Read the model definition and answer for the solid it produces. Units are mm, in the model's axes. A direction names the side the tool comes from. Round coordinates to 2 decimals unless told otherwise and drop trailing zeros. Order: outer loops, then holes, each group sorted by start corner. A loop starts at its lowest first (then second) coordinate and runs counter-clockwise, first axis right, second up. Notation, with made-up numbers: (22, 9) -> (33, 9) arc R24 ccw to (33, 38) -> close; hole circle Ø5 at (66.25, 17). An arc over 180 degrees is marked (long way). Use a Markdown table: item, result. Add a question column.
1. For faces 4 (the face through (0.99, -9.87, 31.18)), 5 (the face through (20, -24, 28)), 6 (the face through (47, -25, 6)), determine the directions among +Z, -Z, +X, -X, +Y, -Y from which every point of the face is accessible in a straight line to the end or side of a thin tool.
2. Consider L1, parallel to Z at x = 1.45, y = -11.5; L2, parallel to Z at x = 48.6, y = -11.5; L3, parallel to Z at x = 1.6, y = -16.5. Determine where each line is inside the solid, lowest interval first. Write a range as [from, to].
3. Section D-D, the plane x = 25 is taken. Give the vertices of the cut face in (y, z).
4. Section A-A, the plane x = 18 is taken. Give the vertices of the cut face in (y, z).
5. Section C-C, the plane y = -14.25 is taken. Give the vertices of the cut face in (x, z), then the cut area to 3 significant figures.
6. The mould has two halves that part along Z. Classify faces 1 (the face through (50, -12, 28)), 2 (the face through (19.01, -24.99, 27.39)), 3 (the face through (16, -25, 0)): +Z half, -Z half, draft (parallel to the pull), parting line (faces both ways), or undercut.
7. Given pin 1 (1.7 mm diameter, centred on x = 20.05, z = 33.45, fed in from +Y); pin 2 (3.5 mm diameter, centred on y = -16.5, z = 4.5, fed in from +X); pin 3 (1.5 mm diameter, centred on y = -17.5, z = 21, fed in from -X); pin 4 (3.5 mm diameter, centred on x = 25, z = 28.5, fed in from +Y), each flat-ended and moving along its own axis, determine where each tip first touches the part or whether it passes through.
8. Section B-B, the plane z = 14.5 is taken. Give the vertices of the cut face in (x, y).
```python
from build123d import *

# Parameters (mm, degrees)
EXTRUDE_1_DEPTH     = 57
SKETCH_2_R          = 7.5
SKETCH_2_R_2        = 1.5
CUT_EXTRUDE_1_DEPTH = 27
SKETCH_3_R          = 1.5
CUT_EXTRUDE_2_DEPTH = 10
SKETCH_4_R          = 1.5
SKETCH_4_R_2        = 3
SKETCH_4_R_3        = 0.75
CUT_EXTRUDE_3_DEPTH = 10
SKETCH_5_R          = 1.5
CUT_EXTRUDE_4_DEPTH = 3
FILLET_2_R          = 2
SKETCH_6_W          = 3
SKETCH_6_H          = 8
CUT_EXTRUDE_5_DEPTH = 44
FILLET_3_R          = 5


with BuildPart() as part:
    # 草图1 → 凸台-拉伸1 (new body)
    with BuildSketch(Plane.XY):
        Polygon((0, 0), (0, -26), (50, -26), (50, 0), (48, 0), (48, -24), (2, -24), (2, 0), align=None)
    extrude(amount=EXTRUDE_1_DEPTH)

    # 草图2 → 切除-拉伸1 (cut)
    with BuildSketch(Plane.ZY):
        with Locations(Location((38.5, -11.5, 0), (0, 0, 270))):
            Circle(SKETCH_2_R)
        with Locations(Location((14.5, -11.5, 0), (0, 0, 270))):
            Circle(SKETCH_2_R_2)
    extrude(amount=-CUT_EXTRUDE_1_DEPTH, mode=Mode.SUBTRACT)

    # 草图3 → 切除-拉伸2 (cut)
    with BuildSketch(Plane(origin=(2, 0, 0), x_dir=(0, 0, -1), z_dir=(1, 0, 0))):
        with Locations(Location((-4.5, -6.5, 0), (0, 0, 90))):
            Circle(SKETCH_3_R)
        with Locations(Location((-4.5, -16.5, 0), (0, 0, 90))):
            Circle(SKETCH_3_R)
        with Locations(Location((-52.5, -16.5, 0), (0, 0, 90))):
            Circle(SKETCH_3_R)
        with Locations(Location((-52.5, -6.5, 0), (0, 0, 90))):
            Circle(SKETCH_3_R)
    extrude(amount=-CUT_EXTRUDE_2_DEPTH, mode=Mode.SUBTRACT)

    # 草图4 → 切除-拉伸3 (cut)
    with BuildSketch(Plane(origin=(0, -24, 0), x_dir=(1, 0, 0), z_dir=(0, 1, 0))):
        with Locations(Location((18, -28.5, 0), (0, 0, 270))):
            Circle(SKETCH_4_R)
        with Locations(Location((25, -21.5, 0), (0, 0, 270))):
            Circle(SKETCH_4_R)
        with Locations(Location((32, -28.5, 0), (0, 0, 270))):
            Circle(SKETCH_4_R)
        with Locations(Location((25, -35.5, 0), (0, 0, 270))):
            Circle(SKETCH_4_R)
        with Locations(Location((25, -28.5, 0), (0, 0, 270))):
            Circle(SKETCH_4_R_2)
        with Locations(Location((20.050252532, -23.550252532, 0), (0, 0, 270))):
            Circle(SKETCH_4_R_3)
        with Locations(Location((29.949747468, -23.550252532, 0), (0, 0, 270))):
            Circle(SKETCH_4_R_3)
        with Locations(Location((29.949747468, -33.449747468, 0), (0, 0, 270))):
            Circle(SKETCH_4_R_3)
        with Locations(Location((20.050252532, -33.449747468, 0), (0, 0, 270))):
            Circle(SKETCH_4_R_3)
    extrude(amount=-CUT_EXTRUDE_3_DEPTH, mode=Mode.SUBTRACT)

    # 草图5 → 切除-拉伸4 (cut)
    with BuildSketch(Plane.ZY.offset(-48)):
        with Locations(Location((14.5, -11.5, 0), (0, 0, 270))):
            Circle(SKETCH_5_R)
        with Locations(Location((38.5, -11.5, 0), (0, 0, 270))):
            Circle(SKETCH_5_R)
    extrude(amount=-CUT_EXTRUDE_4_DEPTH, mode=Mode.SUBTRACT)

    # 圆角2
    fillet_2_edges = [part.edges().sort_by_distance(p)[0] for p in [
        (50, -26, 28.5),
        (0, -26, 28.5),
    ]]
    fillet(fillet_2_edges, radius=FILLET_2_R)

    # 草图6 → 切除-拉伸5 (cut)
    with BuildSketch(Plane.XZ.offset(26)):
        with Locations((48.5, 53)):
            Rectangle(SKETCH_6_W, SKETCH_6_H)
        with Locations((48.5, 4)):
            Rectangle(SKETCH_6_W, SKETCH_6_H)
    extrude(amount=-CUT_EXTRUDE_5_DEPTH, mode=Mode.SUBTRACT)

    # 圆角3
    fillet_3_edges = [part.edges().sort_by_distance(p)[0] for p in [
        (1, 0, 0),
        (47, -25, 57),
        (49, 0, 49),
        (47, -25, 0),
        (49, 0, 8),
        (1, 0, 57),
    ]]
    fillet(fillet_3_edges, radius=FILLET_3_R)


solid = part.part
```
Verdict:
| question | item | result |
|---|---|---|
| 1 | face 4 | -X |
| 1 | face 5 | +Z, -Z, +Y |
| 1 | face 6 | -Z, +X, +Y, -Y |
| 2 | L1 | z = [0, 13], [16, 31], [46, 57] |
| 2 | L2 | z = [8, 13], [16, 37], [40, 49] |
| 2 | L3 | z = [0, 3], [6, 32.91], [44.09, 51], [54, 57] |
| 3 | outline | (-26, 0) -> (-24, 0) -> (-24, 20) -> (-26, 20) -> close; (-26, 23) -> (-24, 23) -> (-24, 25.5) -> (-26, 25.5) -> close; (-26, 31.5) -> (-24, 31.5) -> (-24, 34) -> (-26, 34) -> close; (-26, 37) -> (-24, 37) -> (-24, 57) -> (-26, 57) -> close |
| 4 | outline | (-26, 0) -> (-24, 0) -> (-24, 27) -> (-26, 27) -> close; (-26, 30) -> (-24, 30) -> (-24, 57) -> (-26, 57) -> close |
| 5 | outline | (0, 0) -> (2, 0) -> (2, 31.52) -> (0, 31.52) -> close; (0, 45.48) -> (2, 45.48) -> (2, 57) -> (0, 57) -> close; (48, 8) -> (50, 8) -> (50, 49) -> (48, 49) -> close |
| 5 | area | 168 mm2 |
| 6 | face 1 | draft |
| 6 | face 2 | undercut |
| 6 | face 3 | -Z half |
| 7 | pin 1 | stops at y = -24 |
| 7 | pin 2 | stops at x = 2 |
| 7 | pin 3 | stops at x = 0 |
| 7 | pin 4 | passes through |
| 8 | outline | (0, -24) arc R2 ccw to (2, -26) -> (48, -26) arc R2 ccw to (50, -24) -> (50, -13) -> (48, -13) -> (48, -24) -> (2, -24) -> (2, -13) -> (0, -13) -> close; (0, -10) -> (2, -10) -> (2, 0) -> (0, 0) -> close; (48, -10) -> (50, -10) -> (50, 0) -> (48, 0) -> close |
